```python
from build123d import *

# Parameters (mm, degrees)
F0_W     = 609.6
F0_H     = 438.15
F1_DEPTH = 9.525
F2_W     = 19.05
F2_H     = 876.3
F3_DEPTH = 12.7
F4_W     = 571.5
F4_H     = 19.05
F5_DEPTH = 6.35
F6_W     = 88.9
F6_H     = 101.6
F7_DEPTH = 19.051


with BuildPart() as f1:
    # F0 (on Front) → F1 (new body, symmetric)
    with BuildSketch(Plane.XZ):
        with Locations((56.8960046741, 219.075)):
            Rectangle(F0_W, F0_H)
        with Locations((56.8960046741, -219.075)):
            Rectangle(F0_W, F0_H)
    extrude(amount=F1_DEPTH, both=True)

    # F2 (on face) → F3 (cut)
    with BuildSketch(Plane(origin=(0, 9.525, 0), x_dir=(-1, 0, 0), z_dir=(0, 1, 0))):
        with Locations((-352.1710046741, 0)):
            Rectangle(F2_W, F2_H)
        with Locations((238.3789953259, 0)):
            Rectangle(F2_W, F2_H)
    extrude(amount=-F3_DEPTH, mode=Mode.SUBTRACT)

    # F4 (on face) → F5 (cut)
    with BuildSketch(Plane(origin=(0, 9.525, 0), x_dir=(-1, 0, 0), z_dir=(0, 1, 0))):
        with Locations((-56.8960046741, 309.5625)):
            Rectangle(F4_W, F4_H)
    extrude(amount=-F5_DEPTH, mode=Mode.SUBTRACT)

    # F6 (on face) → F7 (cut, through all)
    with BuildSketch(Plane.XZ.offset(9.525)):
        with Locations((317.2460046741, 387.35)):
            Rectangle(F6_W, F6_H)
    extrude(amount=-F7_DEPTH, mode=Mode.SUBTRACT)


solid = f1.part
```
CAD build for the part. Positions are in the model's coordinates, mm. A direction names the side the tool comes from. Round coordinates to 2 decimals unless told otherwise and drop trailing zeros. Write each loop counter-clockwise with the first axis right and the second up, starting at its lowest first coordinate (ties: lowest second). Pieces come first, ordered by that corner, then holes. Notation, with made-up numbers: M -7,-28.75 L 7,-28.75 A25 cw 7,-8.75 Z; hole C 49,42 d4. An arc over 180 degrees is marked long. One line per question, with ' | ' between items.
1. Pin check, flat tips, straight feed: pin 1 Ø1.5 at (y, z) = (7.5, -21.5) entering from +X; pin 2 Ø5.5 at (y, z) = (-2.5, 408) entering from +X; pin 3 Ø5 at (y, z) = (7, -254.5) entering from -X. Stop position of each tip, or through.
Working result:
pin 1: x = 342.65 | pin 2: x = 272.8 | pin 3: x = -228.85
2. Which spindle directions (+Z, -Z, +X, -X, +Y, -Y) get a long thin tool onto all of the face, cutting with end or side? Do faces 1 (the flat face through (272.796, 0, 387)), 2 (the flat face through (53, 9.525, 379)), 3 (the flat face through (352, -3.175, -45)). Say none if no direction does.
Working result:
face 1: +Z, +X, +Y, -Y | face 2: +Z, -Z, +X, -X, +Y | face 3: +Z, -Z, +X, +Y
3. Mould opens along Z. For faces 4 (the flat face through (53, 0, -438.15)), 5 (the flat face through (-238, -3.175, 6)), 6 (the flat face through (307, 0, 336.55)), 7 (the flat face through (61, 3.175, 310)) say: pulls with the +Z half, pulls with the -Z half, needs draft (parallel to the pull), parting line crosses it, or undercut.
Working result:
face 4: pulls with the -Z half | face 5: needs draft | face 6: pulls with the +Z half | face 7: undercut
4. Cut at C-C on z = 368. Write the cut outline in (x, y) (3 decimals).
Working result:
outline: M -247.904,-9.525 L 272.796,-9.525 L 272.796,9.525 L -228.854,9.525 L -228.854,-3.175 L -247.904,-3.175 Z
5. Cut at A-A on z = -317. Write the cut outline in (x, y) (3 decimals), and give its area (3 significant figures).
Working result:
outline: M -247.904,-9.525 L 361.696,-9.525 L 361.696,-3.175 L 342.646,-3.175 L 342.646,9.525 L -228.854,9.525 L -228.854,-3.175 L -247.904,-3.175 Z | area: 11,100 mm2
6. Probe L1, parallel to Z at x = 123, y = 8; L2, parallel to X at y = 5.75, z = -68.5; L3, parallel to Z at x = 305, y = 1. List the from-to ranges inside material, lowest first. Write a range as from..to.
Working result:
L1: -438.15..300.04, 319.09..438.15 | L2: -228.85..342.65 | L3: -438.15..336.55
7. Cut at B-B on y = -6.5. Write the cut outline in (x, z), and give its area (3 significant figures).
Working result:
outline: M -247.9,-438.15 L 361.7,-438.15 L 361.7,336.55 L 272.8,336.55 L 272.8,438.15 L -247.9,438.15 Z | area: 525,000 mm2
